The model under review builds one solid part; all positions refer to its coordinate system, in mm. A direction names the side the tool comes from. Give positions to 0.01 mm unless a question says otherwise; leave off trailing zeros. Write each loop counter-clockwise with the first axis right and the second up, starting at its lowest first coordinate (ties: lowest second). Pieces come first, ordered by that corner, then holes. Notation, with made-up numbers: (89, 74.5) -> (148, 74.5) arc R28 cw to (148, 111.5) -> close; hole circle Ø7 at (-13.75, -7.5). An arc over 180 degrees is marked (long way). Use CSV: the item, a comma, the result in double quotes.
```python
from build123d import *

# Parameters (mm, degrees)
CROQUIS4_W                = 13
CROQUIS4_H                = 11.3
SALIENTE_EXTRUIR1_DEPTH   = 161
CROQUIS5_W                = 151
CROQUIS5_H                = 3.5
CORTAR_EXTRUIR1_DEPTH     = 6.3
SALIENTE_EXTRUIR3_DEPTH   = 8
CROQUIS9_R                = 2.5
CORTAR_EXTRUIR3_DEPTH     = 179.518038304
SIMETR_A8_COPY_1_DEPTH    = 8
SIMETR_A8_COPY_2_SKETCH_R = 2.5
SIMETR_A8_COPY_2_DEPTH    = 179.518038304
CROQUIS10_R               = 2.5
CORTAR_EXTRUIR4_DEPTH     = 179.518038304
MATRIZL1_COUNT            = 3
MATRIZL1_PITCH            = 40.5


with BuildPart() as part:
    # Barrer1: sweep along a path in Croquis3
    with BuildLine(Plane(origin=(0, 0, 0), x_dir=(1, 0, 0), z_dir=(0, 1, 0))) as barrer1_path:
        Line((0, 0), (0, -37))
    # Croquis1 → Barrer1 (sweep)
    with BuildSketch(Plane.XY):
        Polygon((0, 0), (0, 11.3), (13, 11.3), (13, 6.3), (5, 6.3), (5, 0), align=None)
    barrer1 = sweep(path=barrer1_path.line)

    # Croquis4 → Saliente-Extruir1 (add)
    with BuildSketch(Plane.ZY):
        with Locations((43.5, 5.65)):
            Rectangle(CROQUIS4_W, CROQUIS4_H)
    extrude(amount=-SALIENTE_EXTRUIR1_DEPTH)

    # Simetría5: Barrer1 across plane
    add(barrer1.mirror(Plane.ZY.offset(-80.5)))

    # Croquis5 → Cortar-Extruir1 (cut)
    with BuildSketch(Plane.XZ):
        with Locations((80.5, 38.75)):
            Rectangle(CROQUIS5_W, CROQUIS5_H)
    extrude(amount=-CORTAR_EXTRUIR1_DEPTH, mode=Mode.SUBTRACT)

    # Croquis8 → Saliente-Extruir3 (add)
    with BuildSketch(Plane.XZ):
        with BuildLine():
            Line((161, 46), (165, 46))
            ThreePointArc((165, 46), (171, 40), (165, 34))
            Line((165, 34), (161, 34))
            Line((161, 34), (161, 46))
        make_face()
    saliente_extruir3 = extrude(amount=-SALIENTE_EXTRUIR3_DEPTH)

    # Croquis9 → Cortar-Extruir3 (cut, through all)
    with BuildSketch(Plane.XZ):
        with Locations((165, 40)):
            Circle(CROQUIS9_R)
    cortar_extruir3 = extrude(amount=-CORTAR_EXTRUIR3_DEPTH, mode=Mode.SUBTRACT)

    # Simetría7: Saliente-Extruir3, Cortar-Extruir3 across plane
    add(saliente_extruir3.mirror(Plane(origin=(0, 0, 24), x_dir=(1, 0, 0), z_dir=(0, 0, -1))))
    add(cortar_extruir3.mirror(Plane(origin=(0, 0, 24), x_dir=(1, 0, 0), z_dir=(0, 0, -1))), mode=Mode.SUBTRACT)

    # Simetría8: Saliente-Extruir3, Cortar-Extruir3 across plane
    add(saliente_extruir3.mirror(Plane.ZY.offset(-80.5)))
    add(cortar_extruir3.mirror(Plane.ZY.offset(-80.5)), mode=Mode.SUBTRACT)

    # Simetría8 copy 1 sketch → Simetría8 copy 1 (add)
    with BuildSketch(Plane(origin=(161, 0, 48), x_dir=(-1, 0, 0), z_dir=(0, -1, 0))):
        with BuildLine():
            Line((161, 46), (165, 46))
            ThreePointArc((165, 46), (171, 40), (165, 34))
            Line((165, 34), (161, 34))
            Line((161, 34), (161, 46))
        make_face()
    extrude(amount=-SIMETR_A8_COPY_1_DEPTH)

    # Simetría8 copy 2 sketch → Simetría8 copy 2 (cut, through all)
    with BuildSketch(Plane(origin=(161, 0, 48), x_dir=(-1, 0, 0), z_dir=(0, -1, 0))):
        with Locations((165, 40)):
            Circle(SIMETR_A8_COPY_2_SKETCH_R)
    extrude(amount=-SIMETR_A8_COPY_2_DEPTH, mode=Mode.SUBTRACT)

    # Croquis10 → Cortar-Extruir4 (cut, through all)
    with BuildSketch(Plane(origin=(0, 11.3, 0), x_dir=(1, 0, 0), z_dir=(0, 1, 0))):
        with Locations(Location((121, -45.25, 0), (0, 0, 270))):
            Circle(CROQUIS10_R)
    cortar_extruir4 = extrude(amount=-CORTAR_EXTRUIR4_DEPTH, mode=Mode.SUBTRACT)

    # MatrizL1: Cortar-Extruir4 ×3
    with Locations(*[(-i * MATRIZL1_PITCH, 0, 0) for i in range(1, MATRIZL1_COUNT)]):
        add(cortar_extruir4, mode=Mode.SUBTRACT)


solid = part.part
```
Q1. Consider section B-B (z = 8). Write out the cut boundary in (x, y), then the cut area to 3 significant figures.
Derived:
outline,"(-10, 0) -> (-6.5, 0) -> (-6.5, 8) -> (-10, 8) -> close; (-1.5, 0) -> (5, 0) -> (5, 6.3) -> (13, 6.3) -> (13, 11.3) -> (0, 11.3) -> (0, 8) -> (-1.5, 8) -> close; (148, 6.3) -> (156, 6.3) -> (156, 0) -> (162.5, 0) -> (162.5, 8) -> (161, 8) -> (161, 11.3) -> (148, 11.3) -> close; (167.5, 0) -> (171, 0) -> (171, 8) -> (167.5, 8) -> close"
area,"273 mm2"
Q2. Consider section D-D (x = 104). Write out the cut boundary in (y, z), then the cut area to 3 significant figures.
Derived:
outline,"(0, 40.5) -> (6.3, 40.5) -> (6.3, 37) -> (11.3, 37) -> (11.3, 50) -> (0, 50) -> close"
area,"125 mm2"
Q3. Consider section A-A (x = 80.5). Write out the cut boundary in (y, z), then the cut area to 4 significant figures.
Derived:
outline,"(0, 40.5) -> (6.3, 40.5) -> (6.3, 37) -> (11.3, 37) -> (11.3, 42.75) -> (0, 42.75) -> close; (0, 47.75) -> (11.3, 47.75) -> (11.3, 50) -> (0, 50) -> close"
area,"68.35 mm2"
Q4. Insertion check: pin 1 (12 mm diameter, centred on x = 29.5, z = 37.5, fed in from -Y); pin 2 (5 mm diameter, centred on x = 167, z = 7.5, fed in from +Y); pin 3 (3 mm diameter, centred on x = -3, y = 4, fed in from +Z); pin 4 (2 mm diameter, centred on y = 3.5, z = 22, fed in from +X). Each pin has a flat end and moves straight along its axis. Give the tip position at first contact, or say it passes through.
Derived:
pin 1,"stops at y = 0"
pin 2,"stops at y = 8"
pin 3,"stops at z = 46"
pin 4,"stops at x = 161"
Q5. Machinability: for faces 1 (the flat face through (166, 8, 11)), 2 (the flat face through (-2, 4, 2)), 3 (the flat face through (5, 3, 21)), 4 (the flat face through (148, 9, 19)), which of the approach directions +Z, -Z, +X, -X, +Y, -Y give a long, thin tool a straight path to every point of the face, cutting with its end or side? Answer none if there is none.
Derived:
face 1,"+Z, -Z, +X, +Y"
face 2,"-Z, -X, +Y, -Y"
face 3,"-Z, -Y"
face 4,"-Z, +Y, -Y"
Q6. To check wall thickness, follow probe 1 along Z at (x, y) = (165, 3); probe 2 along X at (y, z) = (5.5, 8); probe 3 along X at (y, z) = (2, 30). State the ranges of each line that lie inside material, in increasing order.
Derived:
probe 1,"z = 2 to 5.5, 10.5 to 14, 34 to 37.5, 42.5 to 46"
probe 2,"x = -10 to -6.5, -1.5 to 5, 156 to 162.5, 167.5 to 171"
probe 3,"x = 0 to 5, 156 to 161"
Q7. Consider section C-C (z = 21). Write out the cut boundary in (x, y).
Derived:
outline,"(0, 0) -> (5, 0) -> (5, 6.3) -> (13, 6.3) -> (13, 11.3) -> (0, 11.3) -> close; (148, 6.3) -> (156, 6.3) -> (156, 0) -> (161, 0) -> (161, 11.3) -> (148, 11.3) -> close"
Q8. The part is to be moulded in two halves that separate along Z. For faces 5 (the flat face through (161, 7, 25)), 6 (the flat face through (-2, 4, 46)), 7 (the flat face through (79, 3, 40.5)), say which applies: pulls with the +Z half, pulls with the -Z half, needs draft (parallel to the pull), parting line crosses it, or undercut.
Derived:
face 5,"undercut"
face 6,"pulls with the +Z half"
face 7,"pulls with the -Z half"
